The figure shows three views and two pictorial views of one solid part (mm, origin at its lowest corner). Answer the questions. A direction names the side the tool comes from. Coordinates: 2 decimals unless noted, no trailing zeros. Loops run counter-clockwise (first coordinate to the right, second up) from the corner with the lowest first, then second, coordinate; pieces in that order, holes last. Notation, with made-up numbers: M 69.5,38 L 124.5,38 A20 cw 124.5,42 Z; hole C 2,9.5 d6. An arc over 180 degrees is marked long. Write each question's results on one line, items separated by ' | '.
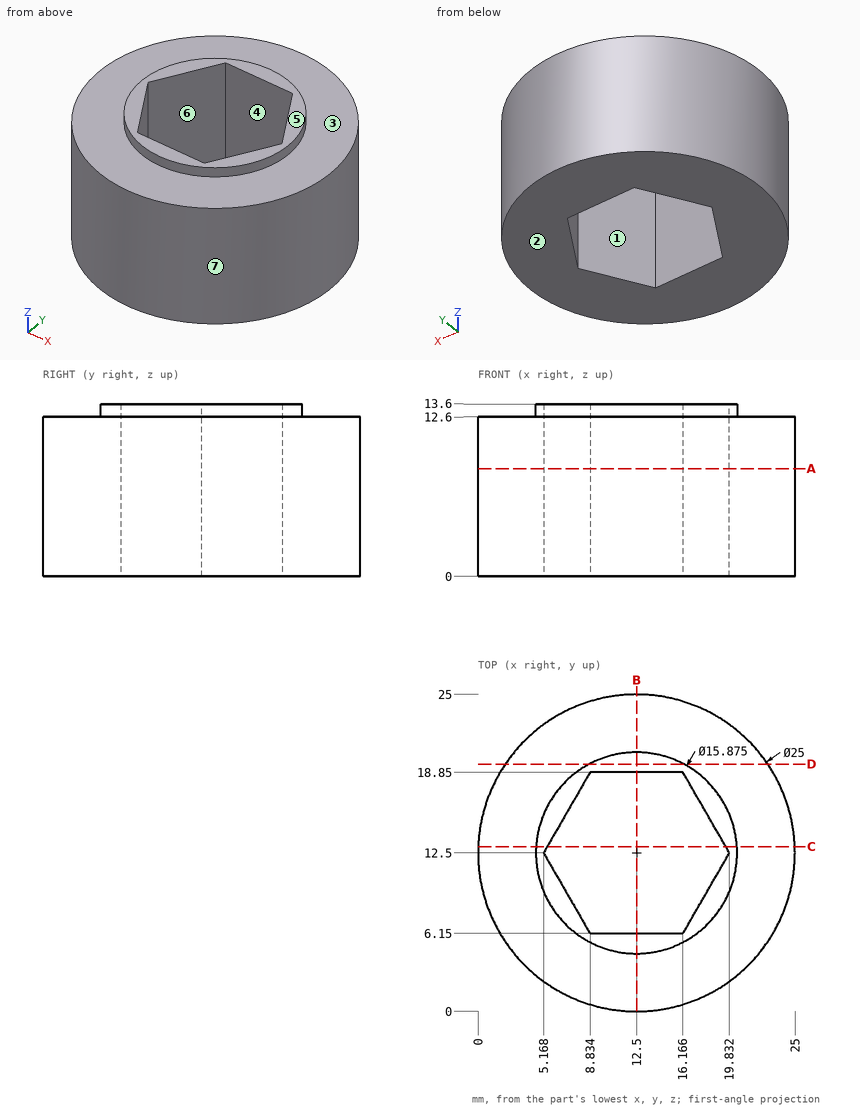
1) Straight lines are drawn through the part: probe 1 along Y at (x, z) = (18, 2.5) (1 decimal); probe 2 along Z at (x, y) = (22.25, 14); probe 3 along Y at (x, z) = (11.25, 8.75). For each, find the intervals that lie inside material, in ascending order. Write a range as [from, to].
Check result:
probe 1: [1.3, 9.3], [15.7, 23.7] | probe 2: [0, 12.6] | probe 3: [0.06, 6.15], [18.85, 24.94]
2) Find section C-C, the plane y = 13. Give the vertices of the cut face in (x, z), and give its area (3 significant figures).
Check result:
outline: M 0.01,0 L 5.46,0 L 5.46,13.6 L 4.58,13.6 L 4.58,12.6 L 0.01,12.6 Z; M 19.54,0 L 24.99,0 L 24.99,12.6 L 20.42,12.6 L 20.42,13.6 L 19.54,13.6 Z | area: 139 mm^2
3) Find section D-D, the plane y = 19.5. Give the vertices of the cut face in (x, z).
Check result:
outline: M 2.14,0 L 22.86,0 L 22.86,12.6 L 16.24,12.6 L 16.24,13.6 L 8.76,13.6 L 8.76,12.6 L 2.14,12.6 Z
4) Given pin 1 Ø6 at (x, z) = (22.5, 5.5) entering from +Y; pin 2 Ø1 at (x, z) = (14, 3) entering from -Y; pin 3 Ø4 at (y, z) = (16, 6.5) entering from -X, each flat-ended and moving along its own axis, determine where each tip first touches the part or whether it passes through.
Check result:
pin 1: y = 22.86 | pin 2: y = 0.04 | pin 3: x = 0.09
5) Find section B-B, the plane x = 12.5. Give the vertices of the cut face in (y, z).
Check result:
outline: M 0,0 L 6.15,0 L 6.15,13.6 L 4.56,13.6 L 4.56,12.6 L 0,12.6 Z; M 18.85,0 L 25,0 L 25,12.6 L 20.44,12.6 L 20.44,13.6 L 18.85,13.6 Z
6) Which of the six approach directions +Z, -Z, +X, -X, +Y, -Y give full straight-line access (tool end or side, diameter ignored) to the marked faces 1, 2 and 3?
Check result:
face 1: +Z, -Z | face 2: -Z, +X, -X, +Y, -Y | face 3: +Z
7) Find section A-A, the plane z = 8.5. Give the vertices of the cut face in (x, y).
Check result:
outline: C 12.5,12.5 d25; hole M 5.17,12.5 L 8.83,6.15 L 16.17,6.15 L 19.83,12.5 L 16.17,18.85 L 8.83,18.85 Z
8) For a pull along Y with two mould halves and no side action, classify the marked faces 4, 5, 6 and 7 as released by +Y, released by -Y, zero draft, split by the parting line, or undercut.
Check result:
face 4: undercut | face 5: zero draft | face 6: undercut | face 7: split by the parting line
